Verification items for this drawing (mm, ordinates from the low corner). A direction names the side the tool comes from. Coordinates: 2 decimals unless noted, no trailing zeros. Loops run counter-clockwise (first coordinate to the right, second up) from the corner with the lowest first, then second, coordinate; pieces in that order, holes last. Notation, with made-up numbers: M 1,-20.5 L 50,-20.5 A26 ccw 50,6.5 Z; hole C 19.25,22 d9. An arc over 180 degrees is marked long. Write each question's results on one line, items separated by ' | '. Start each with the question number.
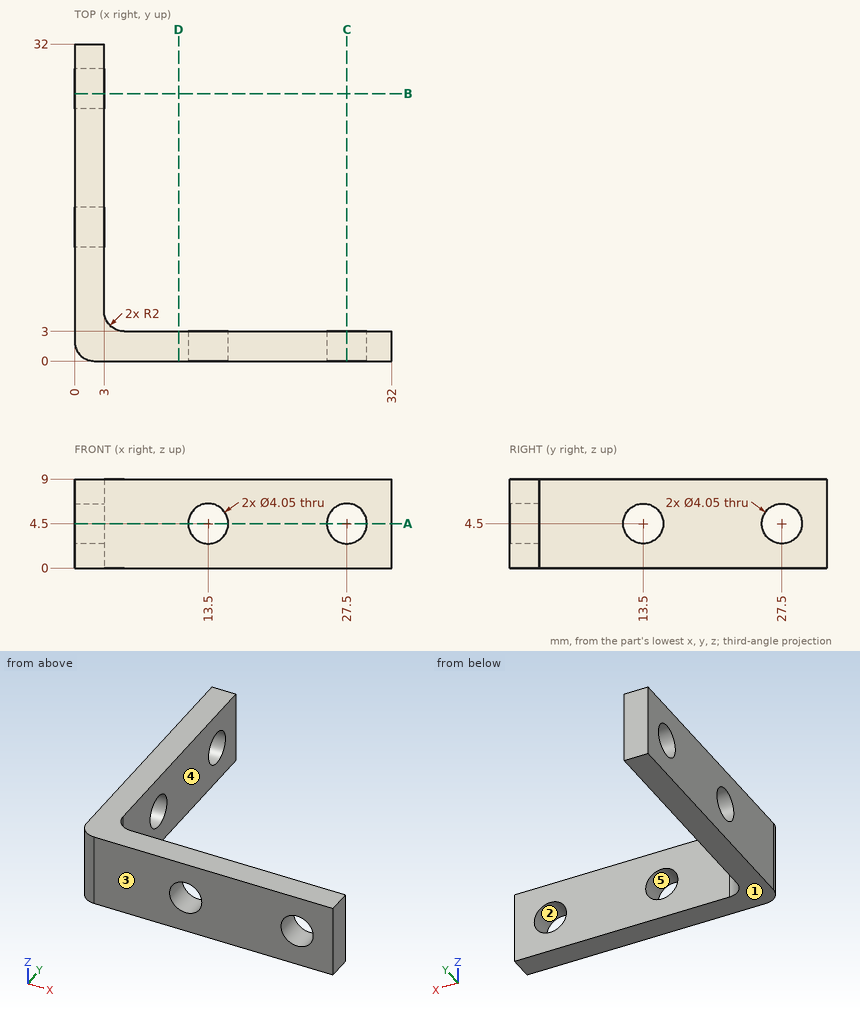
Item 1: Depth check by flat-ended pin: P1, Ø1.5, axis at y = 15.5, z = 6.5, coming from the +X side; P2, Ø2, axis at x = 11, z = 6.5, coming from the +Y side; P3, Ø3.5, axis at y = 13.5, z = 4.5, coming from the +X side. Enter the tip coordinate at first touch or a pass-through.
Item 2: Section check C-C (x = 27.5). Record the cut outline in (y, z) (3 decimals).
Item 3: Section check B-B (y = 27). Record the cut outline in (x, z), plus the area to 3 significant figures.
Item 4: Tool access check on the marked faces 4 and 5. Record the directions out of +Z, -Z, +X, -X, +Y, -Y that give a thin tool (end or side, any length) a straight path to the whole face; none if there is none.
Item 5: Thickness scan on line 1 (Z direction, x = 13.5, y = 2.15) (3 decimals); line 2 (Y direction, x = 2, z = 3); line 3 (Y direction, x = 25.5, z = 5). Record the ranges inside material, lowest first.
Item 6: Release check for a two-part mould opening along Z. For the marked faces 1, 2 and 3 record: +Z half, -Z half, draft (parallel to the pull), parting line (faces both ways), or undercut.
Item 7: Section check D-D (x = 10.5). Record the cut outline in (y, z).
Item 8: Section check A-A (z = 4.5). Record the cut outline in (x, y) (3 decimals).
Computed values:
1) P1: stops at x = 3 | P2: stops at y = 3 | P3: passes through
2) outline: M 0,0 L 3,0 L 3,2.475 L 0,2.475 Z; M 0,6.525 L 3,6.525 L 3,9 L 0,9 Z
3) outline: M 0,0 L 3,0 L 3,2.54 L 0,2.54 Z; M 0,6.46 L 3,6.46 L 3,9 L 0,9 Z | area: 15.2 mm²
4) face 4: +Z, -Z, +X, +Y | face 5: +Y, -Y
5) line 1: z = 0 to 2.475, 6.525 to 9 | line 2: y = 0 to 12.14, 14.86 to 26.14, 28.86 to 32 | line 3: y = 0 to 3
6) face 1: -Z half | face 2: undercut | face 3: draft
7) outline: M 0,0 L 3,0 L 3,9 L 0,9 Z
8) outline: M 0,2 A2 ccw 2,0 L 11.475,0 L 11.475,3 L 5,3 A2 cw 3,5 L 3,11.475 L 0,11.475 Z; M 0,15.525 L 3,15.525 L 3,25.475 L 0,25.475 Z; M 0,29.525 L 3,29.525 L 3,32 L 0,32 Z; M 15.525,0 L 25.475,0 L 25.475,3 L 15.525,3 Z; M 29.525,0 L 32,0 L 32,3 L 29.525,3 Z
